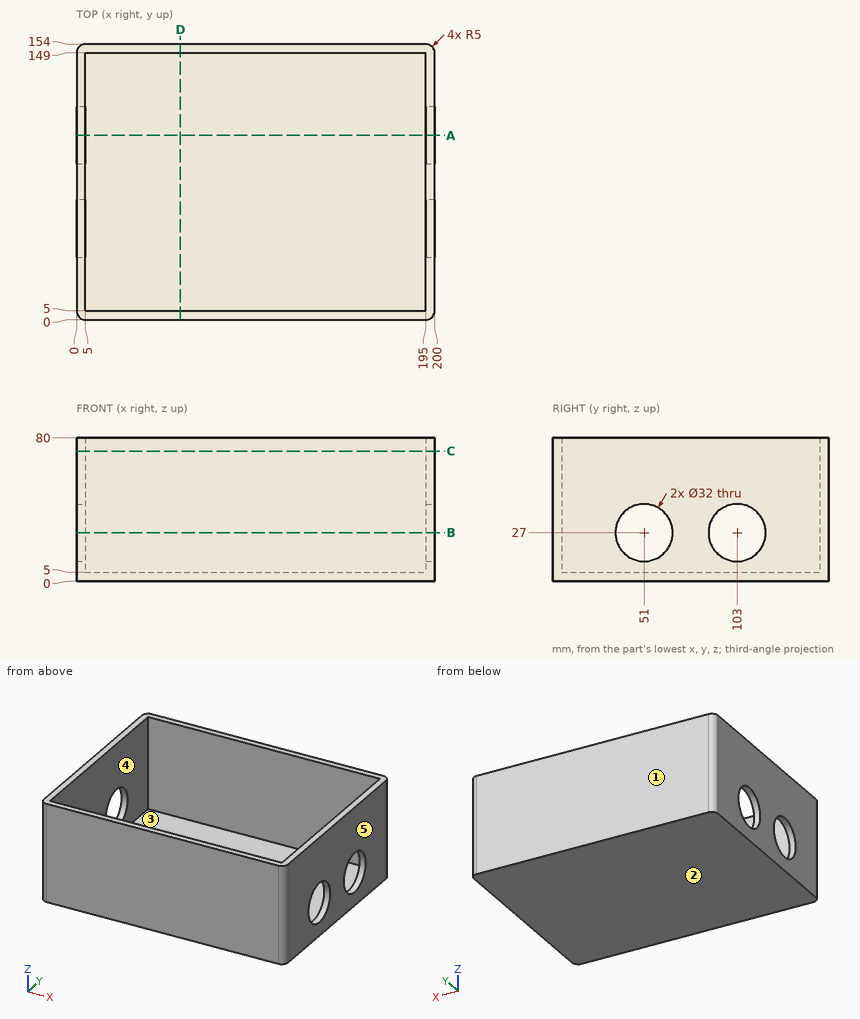
Input: dimensioned drawing with shaded views. Units: mm. Origin: part minimum x, y, z. A direction names the side the tool comes from. Coordinates: 2 decimals unless noted, no trailing zeros. Order: outer loops, then holes, each group sorted by start corner. A loop starts at its lowest first (then second) coordinate and runs counter-clockwise, first axis right, second up.
Item 1: Draft query along Y for the marked faces 1, 2 and 3. Return one class per face: released by +Y, released by -Y, zero draft, split by the parting line, or undercut.
Answer:
face 1: released by +Y
face 2: zero draft
face 3: undercut
Item 2: Section query A-A (y = 103). Output: boundary loops of the cut face in (x, z), then the cut area to 3 significant figures.
Answer:
outline: (0, 0) - (200, 0) - (200, 11) - (195, 11) - (195, 5) - (5, 5) - (5, 11) - (0, 11) - close; (0, 43) - (5, 43) - (5, 80) - (0, 80) - close; (195, 43) - (200, 43) - (200, 80) - (195, 80) - close
area: 1,430 mm2
Item 3: Contact query for flat-ended pins moving along their axis: P1, Ø12, axis at y = 91.5, z = 29, coming from the +X side; P2, Ø2, axis at x = 93.5, y = 65.5, coming from the +Z side. Output: stop coordinate, or through.
Answer:
P1: stops at x = 200
P2: stops at z = 5
Item 4: Section query B-B (z = 27). Output: boundary loops of the cut face in (x, y), then the cut area to 3 significant figures.
Answer:
outline: (0, 5) arc R5 ccw to (5, 0) - (195, 0) arc R5 ccw to (200, 5) - (200, 35) - (195, 35) - (195, 5) - (5, 5) - (5, 35) - (0, 35) - close; (0, 67) - (5, 67) - (5, 87) - (0, 87) - close; (0, 119) - (5, 119) - (5, 149) - (195, 149) - (195, 119) - (200, 119) - (200, 149) arc R5 ccw to (195, 154) - (5, 154) arc R5 ccw to (0, 149) - close; (195, 67) - (200, 67) - (200, 87) - (195, 87) - close
area: 2,780 mm2
Item 5: Access query for the marked faces 4 and 5. Directions: +Z, -Z, +X, -X, +Y, -Y. A direction counts if a zero-diameter tool reaches every point of the face in a straight line with its end or side. Return the directions, or none.
Answer:
face 4: +Z
face 5: +Z, -Z, +X, +Y, -Y
Item 6: Section query C-C (z = 72.5). Output: boundary loops of the cut face in (x, y), then the cut area to 3 significant figures.
Answer:
outline: (0, 5) arc R5 ccw to (5, 0) - (195, 0) arc R5 ccw to (200, 5) - (200, 149) arc R5 ccw to (195, 154) - (5, 154) arc R5 ccw to (0, 149) - close; hole (5, 5) - (195, 5) - (195, 149) - (5, 149) - close
area: 3,420 mm2
Item 7: Section query D-D (x = 58). Output: boundary loops of the cut face in (y, z), then the cut area to 3 significant figures.
Answer:
outline: (0, 0) - (154, 0) - (154, 80) - (149, 80) - (149, 5) - (5, 5) - (5, 80) - (0, 80) - close
area: 1,520 mm2
Item 8: Material intervals for line 1 along Y through (x, z) = (11.5, 32.5); line 2 along X through (y, z) = (40, 50); line 3 along Z through (x, y) = (198.9, 103), sorted ascending.
Answer:
line 1: y = 0 to 5, 149 to 154
line 2: x = 0 to 5, 195 to 200
line 3: z = 0 to 11, 43 to 80
